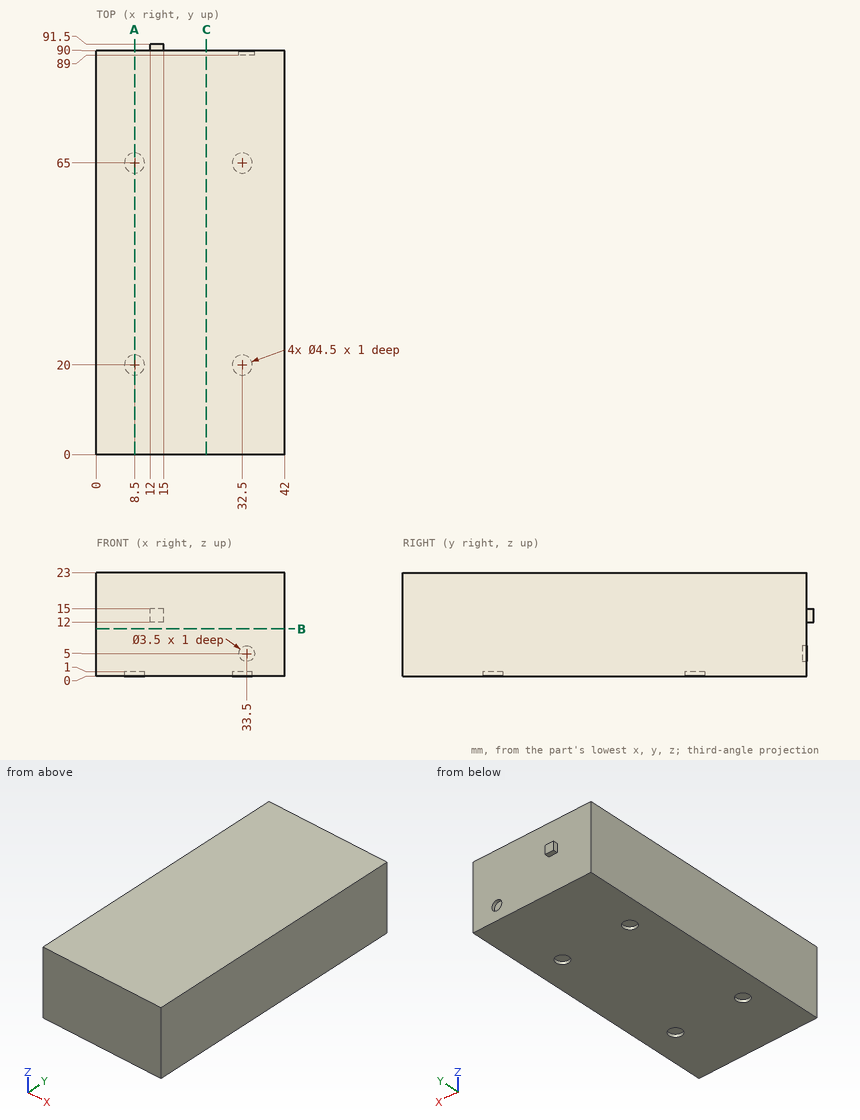
Input: dimensioned drawing with shaded views. Units: mm. Origin: part minimum x, y, z. Coordinates: 2 decimals unless noted, no trailing zeros. Loops run counter-clockwise (first coordinate to the right, second up) from the corner with the lowest first, then second, coordinate; pieces in that order, holes last. Notation, with made-up numbers: M 68.5,-21 L 74.5,-21 A16 ccw 74.5,-9 Z; hole C 29,22.5 d11. An arc over 180 degrees is marked long. One line per item, written item: value. Start each with the question number.
1) Material intervals for L1, parallel to X at y = 65, z = 0.35; L2, parallel to Y at x = 8.5, z = 0.6; L3, parallel to X at y = 89.45, z = 5, sorted ascending. Write a range as from..to.
2) Cut plane A-A (x = 8.5). Return loops of the section in (y, z), then the cut area to 3 significant figures.
3) Pin query (flat end, axial travel): P1, Ø6, axis at x = 32.5, y = 65, coming from the -Z side; P2, Ø2.5, axis at x = 8.5, y = 20, coming from the -Z side; P3, Ø0.8, axis at y = 90.5, z = 14, coming from the +X side; P4, Ø0.8, axis at y = 91, z = 14, coming from the -X side. Return the tip coordinate at first contact, or that it passes through.
4) Cut plane B-B (z = 10.5). Return loops of the section in (x, y).
5) Cut plane C-C (x = 24.5). Return loops of the section in (y, z), then the cut area to 3 significant figures.
Evaluation:
1. L1: 0..6.25, 10.75..30.25, 34.75..42
1. L2: 0..17.75, 22.25..62.75, 67.25..90
1. L3: 0..31.75, 35.25..42
2. outline: M 0,0 L 17.75,0 L 17.75,1 L 22.25,1 L 22.25,0 L 62.75,0 L 62.75,1 L 67.25,1 L 67.25,0 L 90,0 L 90,23 L 0,23 Z
2. area: 2,060 mm^2
3. P1: z = 0
3. P2: z = 1
3. P3: x = 15
3. P4: x = 12
4. outline: M 0,0 L 42,0 L 42,90 L 0,90 Z
5. outline: M 0,0 L 90,0 L 90,23 L 0,23 Z
5. area: 2,070 mm^2
